Answer from the drawing. Dimensions are ordinates in mm from the lowest x, y and z of the part. Coordinates: 2 decimals unless noted, no trailing zeros. Write each loop counter-clockwise with the first axis right and the second up, starting at its lowest first coordinate (ties: lowest second). Pieces come first, ordered by that corner, then holes.
(1) Section A-A on x = 49.5 is taken. Write down the section's boundary in (y, z) (1 decimal).
(2) Section B-B on z = 12.5 is taken. Write down the section's boundary in (x, y).
(3) Find the intervals of material crossed by probe 1 along Z at (x, y) = (36.5, 8.25) (1 decimal); probe 2 along Y at (x, z) = (49.5, 148.8); probe 3 along X at (y, z) = (2.25, 40.5), in increasing order.
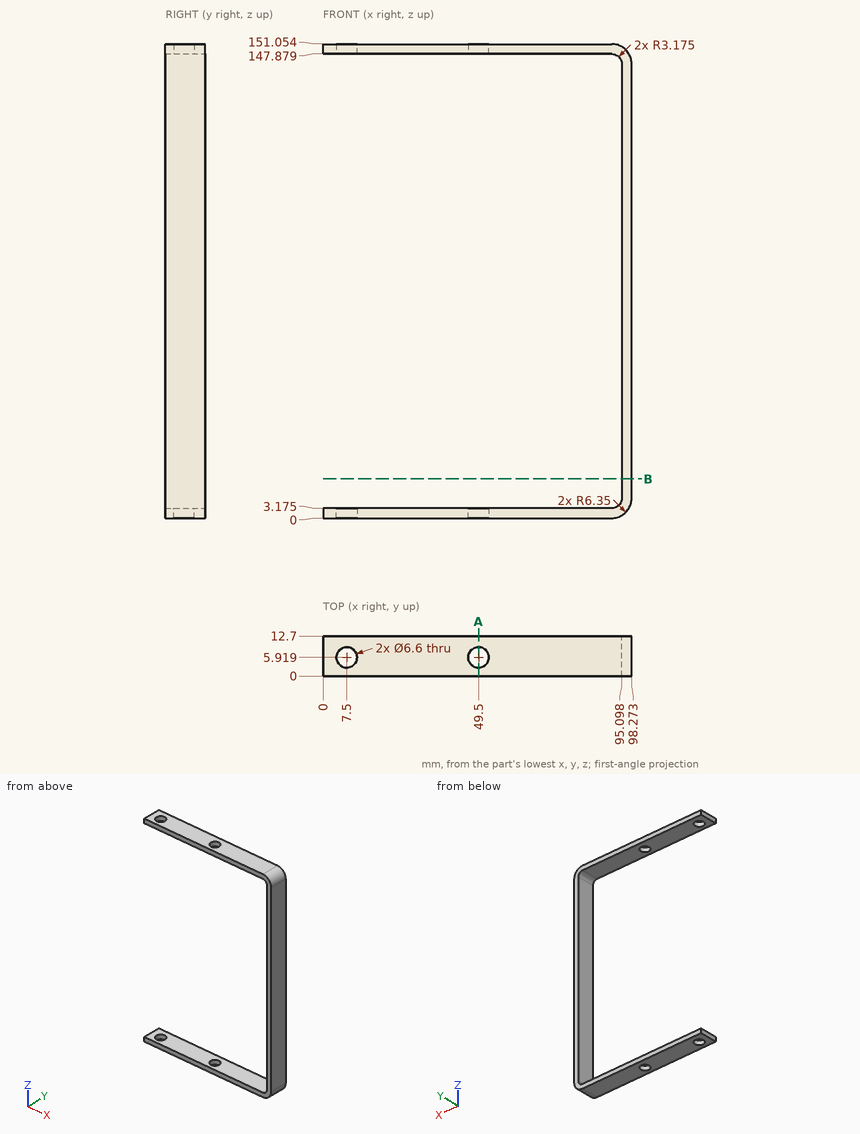
Response:
1. outline: (0, 0) - (2.6, 0) - (2.6, 3.2) - (0, 3.2) - close; (0, 147.9) - (2.6, 147.9) - (2.6, 151.1) - (0, 151.1) - close; (9.2, 0) - (12.7, 0) - (12.7, 3.2) - (9.2, 3.2) - close; (9.2, 147.9) - (12.7, 147.9) - (12.7, 151.1) - (9.2, 151.1) - close
2. outline: (95.1, 0) - (98.27, 0) - (98.27, 12.7) - (95.1, 12.7) - close
3. probe 1: z = 0 to 3.2, 147.9 to 151.1
3. probe 2: y = 0 to 2.62, 9.22 to 12.7
3. probe 3: x = 95.1 to 98.27
